```python
from build123d import *

# Parameters (mm, degrees)
SKETCH1_W                             = 92.75
SKETCH1_H                             = 86.75
SKETCH1_R                             = 1.55
BOSS_EXTRUDE1_FIRST_PCB_DEPTH         = 1.6
SKETCH2_R                             = 6
BOSS_EXTRUDE2_SPEAKER_DEPTH           = 9.5
SKETCH15_R                            = 1.25
CUT_EXTRUDE1_SPEAKER_HOLE_DEPTH       = 5
SKETCH3_W                             = 12
SKETCH3_H                             = 11.65
BOSS_EXTRUDE3_ROTARY_SWITCH_DEPTH     = 4.5
SKETCH4_W                             = 5.83
SKETCH4_H                             = 5.83
BOSS_EXTRUDE4_RESET_SWITCH_DEPTH      = 3.5
SKETCH5_R                             = 1.75
BOSS_EXTRUDE5_RESET_BUTTON_DEPTH      = 0.5
SKETCH16_R                            = 3.415
BOSS_EXTRUDE6_ROTARY_SWITCH_DEPTH     = 7
SKETCH17_R                            = 2.935
BOSS_EXTRUDE7_ROTARY_SWITCH_DEPTH     = 6.4
BOSS_EXTRUDE8_ROTARY_SWITCH_DEPTH     = 6.2
BOSS_EXTRUDE9_SD_CARD_SLOT_DEPTH      = 3
SKETCH19_W                            = 50
SKETCH19_H                            = 2.5
BOSS_EXTRUDE10_CONNECTOR_DEPTH        = 4.2
SKETCH11_W                            = 92.75
SKETCH11_H                            = 70
SKETCH11_R                            = 1.55
BOSS_EXTRUDE11_UPPER_PCB_DEPTH        = 1.6
SKETCH12_W                            = 78.45
SKETCH12_H                            = 51
BOSS_EXTRUDE12_LCD_DEPTH              = 8.3
SKETCH24_W                            = 5.4
SKETCH24_H                            = 43
BOSS_EXTRUDE13_LCD_BUMPOUT_DEPTH      = 3.5
CUT_EXTRUDE2_SCREEN_RECESS_DEPTH      = 1
SKETCH21_W                            = 20.2
SKETCH21_H                            = 8.85
SKETCH21_W_2                          = 18.2
SKETCH21_H_2                          = 6.85
BOSS_EXTRUDE14_CONNECTORS_DEPTH       = 9
SKETCH22_W                            = 18.2
SKETCH22_H                            = 6.85
BOSS_EXTRUDE15_CONNECTOR_RECESS_DEPTH = 2.55
SKETCH23_W                            = 4.4
SKETCH23_H                            = 1
CUT_EXTRUDE3_CONNECTOR_NOTCH_DEPTH    = 6.45
SKETCH20_W                            = 2.153
SKETCH20_H                            = 23.75
BOSS_EXTRUDE16_SD_CARD_DEPTH          = 10.4
FILLET1_SD_CARD_R                     = 1
CROQUIS1_W                            = 18.2
CROQUIS1_H                            = 6.85
SALIENTE_EXTRUIR1_DEPTH               = 15


with BuildPart() as part:
    # Sketch1 → Boss-Extrude1 - First PCB (new body)
    with BuildSketch(Plane.XY):
        Rectangle(SKETCH1_W, SKETCH1_H)
        with Locations((-43.975, 40.975)):
            Circle(SKETCH1_R, mode=Mode.SUBTRACT)
        with Locations((43.975, 40.975)):
            Circle(SKETCH1_R, mode=Mode.SUBTRACT)
        with Locations((43.975, -24.025)):
            Circle(SKETCH1_R, mode=Mode.SUBTRACT)
        with Locations((-43.975, -24.025)):
            Circle(SKETCH1_R, mode=Mode.SUBTRACT)
    extrude(amount=BOSS_EXTRUDE1_FIRST_PCB_DEPTH)

    # Sketch2 → Boss-Extrude2 - Speaker (add)
    with BuildSketch(Plane.XY.offset(1.6)):
        with Locations((18.625, -35.375)):
            Circle(SKETCH2_R)
    extrude(amount=BOSS_EXTRUDE2_SPEAKER_DEPTH)

    # Sketch15 → Cut-Extrude1 - Speaker Hole (cut)
    with BuildSketch(Plane.XY.offset(11.1)):
        with Locations((18.625, -35.375)):
            Circle(SKETCH15_R)
    extrude(amount=-CUT_EXTRUDE1_SPEAKER_HOLE_DEPTH, mode=Mode.SUBTRACT)

    # Sketch3 → Boss-Extrude3 - Rotary Switch (add)
    with BuildSketch(Plane(origin=(0, 0, 1.6), x_dir=(-1, 0, 0), z_dir=(0, 0, 1))):
        with Locations((-36.375, 35.375)):
            Rectangle(SKETCH3_W, SKETCH3_H)
    extrude(amount=BOSS_EXTRUDE3_ROTARY_SWITCH_DEPTH)

    # Sketch4 → Boss-Extrude4 - Reset Switch (add)
    with BuildSketch(Plane(origin=(0, 0, 1.6), x_dir=(-1, 0, 0), z_dir=(0, 0, 1))):
        with Locations((-3.375, 35.375)):
            Rectangle(SKETCH4_W, SKETCH4_H)
    extrude(amount=BOSS_EXTRUDE4_RESET_SWITCH_DEPTH)

    # Sketch5 → Boss-Extrude5 - Reset Button (add)
    with BuildSketch(Plane(origin=(0, 0, 5.1), x_dir=(-1, 0, 0), z_dir=(0, 0, 1))):
        with Locations((-3.375, 35.375)):
            Circle(SKETCH5_R)
    extrude(amount=BOSS_EXTRUDE5_RESET_BUTTON_DEPTH)

    # Sketch16 → Boss-Extrude6 - Rotary Switch (add)
    with BuildSketch(Plane.XY.offset(6.1)):
        with Locations((36.375, -35.375)):
            Circle(SKETCH16_R)
    extrude(amount=BOSS_EXTRUDE6_ROTARY_SWITCH_DEPTH)

    # Sketch17 → Boss-Extrude7 - Rotary Switch (add)
    with BuildSketch(Plane.XY.offset(13.1)):
        with Locations((36.375, -35.375)):
            Circle(SKETCH17_R)
    extrude(amount=BOSS_EXTRUDE7_ROTARY_SWITCH_DEPTH)

    # Sketch18 → Boss-Extrude8 - Rotary Switch (add)
    with BuildSketch(Plane.XY.offset(19.5)):
        with BuildLine():
            Line((33.831773703, -33.91), (38.918226297, -33.91))
            ThreePointArc((38.918226297, -33.91), (36.375, -38.31), (33.831773703, -33.91))
        make_face()
    extrude(amount=BOSS_EXTRUDE8_ROTARY_SWITCH_DEPTH)

    # Sketch9 → Boss-Extrude9 - SD Card Slot (add)
    with BuildSketch(Plane(origin=(0, 0, 0), x_dir=(1, 0, 0), z_dir=(0, 0, -1))):
        Polygon((-46.125, 5.425), (-27.875, 5.425), (-25.875, 3.425), (-20.375, 3.425), (-20.375, -20.975), (-46.125, -20.975), align=None)
    extrude(amount=BOSS_EXTRUDE9_SD_CARD_SLOT_DEPTH)

    # Sketch19 → Boss-Extrude10 - Connector (add)
    with BuildSketch(Plane.XY.offset(1.6)):
        with Locations((-8.375, -24.125)):
            Rectangle(SKETCH19_W, SKETCH19_H)
    extrude(amount=BOSS_EXTRUDE10_CONNECTOR_DEPTH)

    # Sketch11 → Boss-Extrude11 - Upper PCB (add)
    with BuildSketch(Plane(origin=(0, -2, 5.8), x_dir=(1, 0, 0), z_dir=(0, 0, -1))):
        with Locations((0, -10.375)):
            Rectangle(SKETCH11_W, SKETCH11_H)
        with Locations((-43.975, -42.975)):
            Circle(SKETCH11_R, mode=Mode.SUBTRACT)
        with Locations((-43.975, 22.025)):
            Circle(SKETCH11_R, mode=Mode.SUBTRACT)
        with Locations((43.975, -42.975)):
            Circle(SKETCH11_R, mode=Mode.SUBTRACT)
        with Locations((43.975, 22.025)):
            Circle(SKETCH11_R, mode=Mode.SUBTRACT)
    extrude(amount=-BOSS_EXTRUDE11_UPPER_PCB_DEPTH)

    # Sketch12 → Boss-Extrude12 - LCD (add)
    with BuildSketch(Plane(origin=(0, 0, 7.4), x_dir=(-1, 0, 0), z_dir=(0, 0, 1))):
        with Locations((-0.2, -8.475)):
            Rectangle(SKETCH12_W, SKETCH12_H)
    extrude(amount=BOSS_EXTRUDE12_LCD_DEPTH)

    # Sketch24 → Boss-Extrude13 - LCD Bumpout (add)
    with BuildSketch(Plane.XY.offset(7.4)):
        with Locations((-41.725, 7.875)):
            Rectangle(SKETCH24_W, SKETCH24_H)
    extrude(amount=BOSS_EXTRUDE13_LCD_BUMPOUT_DEPTH)

    # Sketch13 → Cut-Extrude2 - Screen Recess (cut)
    with BuildSketch(Plane(origin=(0, 0, 15.7), x_dir=(-1, 0, 0), z_dir=(0, 0, 1))):
        with BuildLine():
            Line((-34.2, 11.525), (33.8, 11.525))
            ThreePointArc((33.8, 11.525), (35.214213562, 10.939213562), (35.8, 9.525))
            Line((35.8, 9.525), (35.8, -26.475))
            ThreePointArc((35.8, -26.475), (35.214213562, -27.889213562), (33.8, -28.475))
            Line((33.8, -28.475), (-34.2, -28.475))
            ThreePointArc((-34.2, -28.475), (-35.614213562, -27.889213562), (-36.2, -26.475))
            Line((-36.2, -26.475), (-36.2, 9.525))
            ThreePointArc((-36.2, 9.525), (-35.614213562, 10.939213562), (-34.2, 11.525))
        make_face()
    extrude(amount=-CUT_EXTRUDE2_SCREEN_RECESS_DEPTH, mode=Mode.SUBTRACT)

    # Sketch21 → Boss-Extrude14 - Connectors (add)
    with BuildSketch(Plane(origin=(0, 0, 0), x_dir=(-1, 0, 0), z_dir=(0, 0, -1))):
        with Locations((-15.525, 32.45)):
            Rectangle(SKETCH21_W, SKETCH21_H)
        with Locations((-15.525, 32.45)):
            Rectangle(SKETCH21_W_2, SKETCH21_H_2, mode=Mode.SUBTRACT)
        with Locations((14.975, 32.45)):
            Rectangle(SKETCH21_W, SKETCH21_H)
        with Locations((14.975, 32.45)):
            Rectangle(SKETCH21_W_2, SKETCH21_H_2, mode=Mode.SUBTRACT)
    extrude(amount=BOSS_EXTRUDE14_CONNECTORS_DEPTH)

    # Sketch22 → Boss-Extrude15 - Connector Recess (add)
    with BuildSketch(Plane(origin=(0, 0, 0), x_dir=(-1, 0, 0), z_dir=(0, 0, -1))):
        with Locations((-15.525, 32.45)):
            Rectangle(SKETCH22_W, SKETCH22_H)
        with Locations((14.975, 32.45)):
            Rectangle(SKETCH22_W, SKETCH22_H)
    extrude(amount=BOSS_EXTRUDE15_CONNECTOR_RECESS_DEPTH)

    # Sketch23 → Cut-Extrude3 - Connector Notch (cut)
    with BuildSketch(Plane(origin=(0, 0, -9), x_dir=(-1, 0, 0), z_dir=(0, 0, -1))):
        with Locations((-15.525, 36.375)):
            Rectangle(SKETCH23_W, SKETCH23_H)
        with Locations((14.975, 36.375)):
            Rectangle(SKETCH23_W, SKETCH23_H)
    extrude(amount=-CUT_EXTRUDE3_CONNECTOR_NOTCH_DEPTH, mode=Mode.SUBTRACT)

    # Sketch20 → Boss-Extrude16 - SD Card (add)
    with BuildSketch(Plane.ZY.offset(46.125)):
        with Locations((-1.3465, 7.775)):
            Rectangle(SKETCH20_W, SKETCH20_H)
    extrude(amount=BOSS_EXTRUDE16_SD_CARD_DEPTH)

    # Fillet1 - SD Card
    fillet1_sd_card_edges = [part.edges().sort_by_distance(p)[0] for p in [
        (-56.525, -4.1, -1.3465),
        (-56.525, 19.65, -1.3465),
    ]]
    fillet(fillet1_sd_card_edges, radius=FILLET1_SD_CARD_R)

    # Croquis1 → Saliente-Extruir1 (add)
    with BuildSketch(Plane(origin=(0, 0, -2.55), x_dir=(-1, 0, 0), z_dir=(0, 0, -1))):
        with Locations((-15.525, 32.45)):
            Rectangle(CROQUIS1_W, CROQUIS1_H)
        with Locations((14.975, 32.45)):
            Rectangle(CROQUIS1_W, CROQUIS1_H)
    extrude(amount=SALIENTE_EXTRUIR1_DEPTH)


solid = part.part
```
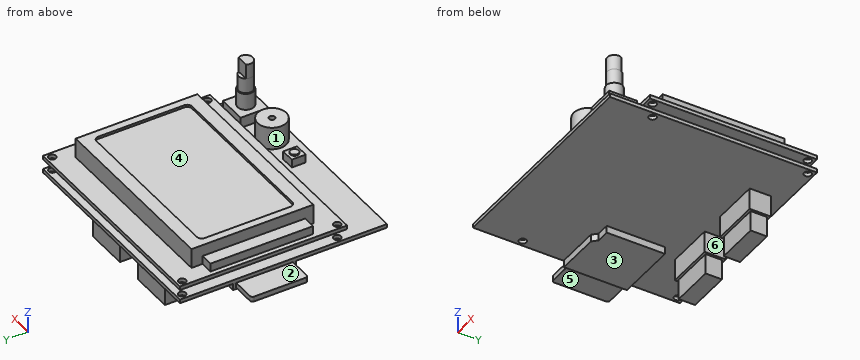
Build history of the part. All positions in model axes, mm. Face numbers are marked on the shaded views. A direction names the side the tool comes from. Round coordinates to 2 decimals unless told otherwise and drop trailing zeros. Order: outer loops, then holes, each group sorted by start corner. A loop starts at its lowest first (then second) coordinate and runs counter-clockwise, first axis right, second up. Notation, with made-up numbers: (36.25, -2.5) -> (72.25, -2.5) arc R26 cw to (72.25, 13.5) -> close; hole circle Ø9 at (78.5, 43). An arc over 180 degrees is marked (long way). Answer in a Markdown table with one row per item.
1) Mould opens along Y. For the marked faces 1 and 2 say: released by +Y, released by -Y, zero draft, split by the parting line, or undercut.
Values:
| item | result |
|---|---|
| face 1 | undercut |
| face 2 | zero draft |
2) Which spindle directions (+Z, -Z, +X, -X, +Y, -Y) get a long thin tool onto all of the face, cutting with end or side? Do the marked faces 3, 4, 5 and 6. Say none if no direction does.
Values:
| item | result |
|---|---|
| face 3 | -Z, +X, -X, -Y |
| face 4 | +Z |
| face 5 | -Z, -X, +Y, -Y |
| face 6 | -Z, +Y, -Y |
3) Band-saw the part on C-C on x = -48. Give the cut face in (y, z), and give its area (3 significant figures).
Values:
| item | result |
|---|---|
| outline | (-4.1, -2.42) -> (19.65, -2.42) -> (19.65, -0.27) -> (-4.1, -0.27) -> close |
| area | 51.1 mm2 |
4) Pin check, flat tips, straight feed: P1, Ø8, axis at y = -28, z = -6.5, coming from the -X side; P2, Ø3, axis at x = -16.5, y = 8.5, coming from the -Z side; P3, Ø6.5, axis at x = 4.5, y = -36.5, coming from the +Z side; P4, Ø4.5, axis at x = 16, z = -2.5, coming from the +Y side (3 decimals). Stop position of each tip, or through.
Values:
| item | result |
|---|---|
| P1 | through |
| P2 | z = 0 |
| P3 | z = 5.6 |
| P4 | y = 36.875 |
5) Wall check: L1, parallel to Z at x = -27, y = 29; L2, parallel to Z at x = 9, y = 19; L3, parallel to X at y = 35, z = -16 (3 decimals). Give the ranges that are in metal, low to high.
Values:
| item | result |
|---|---|
| L1 | 0 to 1.6, 5.8 to 15.7 |
| L2 | 0 to 1.6, 5.8 to 14.7 |
| L3 | -24.075 to -5.875, 6.425 to 24.625 |
6) Band-saw the part on D-D on z = -5.5. Give the cut face in (x, y) (3 decimals), and give its area (3 significant figures).
Values:
| item | result |
|---|---|
| outline | (-25.075, 28.025) -> (-4.875, 28.025) -> (-4.875, 36.875) -> (-12.775, 36.875) -> (-12.775, 35.875) -> (-17.175, 35.875) -> (-17.175, 36.875) -> (-25.075, 36.875) -> close; (5.425, 28.025) -> (25.625, 28.025) -> (25.625, 36.875) -> (17.725, 36.875) -> (17.725, 35.875) -> (13.325, 35.875) -> (13.325, 36.875) -> (5.425, 36.875) -> close |
| area | 349 mm2 |
7) Band-saw the part on B-B on y = 4.5. Give the cut face in (x, z) (3 decimals), and give its area (3 significant figures).
Values:
| item | result |
|---|---|
| outline | (-56.525, -2.423) -> (-46.125, -2.423) -> (-46.125, -3) -> (-20.375, -3) -> (-20.375, 0) -> (46.375, 0) -> (46.375, 1.6) -> (-46.375, 1.6) -> (-46.375, 0) -> (-46.125, 0) -> (-46.125, -0.27) -> (-56.525, -0.27) -> close; (-46.375, 5.8) -> (46.375, 5.8) -> (46.375, 7.4) -> (39.425, 7.4) -> (39.425, 15.7) -> (36.2, 15.7) -> (36.2, 14.7) -> (-35.8, 14.7) -> (-35.8, 15.7) -> (-39.025, 15.7) -> (-39.025, 10.9) -> (-44.425, 10.9) -> (-44.425, 7.4) -> (-46.375, 7.4) -> close |
| area | 994 mm2 |
8) Band-saw the part on A-A on z = -11. Give the cut face in (x, y) (3 decimals), and give its area (3 significant figures).
Values:
| item | result |
|---|---|
| outline | (-24.075, 29.025) -> (-5.875, 29.025) -> (-5.875, 35.875) -> (-24.075, 35.875) -> close; (6.425, 29.025) -> (24.625, 29.025) -> (24.625, 35.875) -> (6.425, 35.875) -> close |
| area | 249 mm2 |
